Design review of the part built by this model. Coordinates are the model's own, in mm. Give positions to 0.01 mm unless a question says otherwise; leave off trailing zeros. Write each loop counter-clockwise with the first axis right and the second up, starting at its lowest first coordinate (ties: lowest second). Pieces come first, ordered by that corner, then holes. Notation, with made-up numbers: (40, 51) -> (61, 51) arc R15 cw to (61, 79) -> close; hole circle Ø6 at (59, 31.5). An arc over 180 degrees is marked (long way). Write each question's results on one line, items separated by ' | '. Start each with the question number.
(1) Take a section at C-C (z = -7). State the section outline as (x, y) points (3 decimals), plus the area to 3 significant figures.
(2) Take a section at A-A (z = 4.5). State the section outline as (x, y) points (3 decimals), plus the area to 3 significant figures.
(3) Clearance check with flat-ended pins moving along their axes: pin 1 (1.5 mm diameter, centred on y = 1.5, z = -0.5, fed in from -X) (3 decimals); pin 2 (1 mm diameter, centred on x = -78.5, y = 2.5, fed in from -Z). State where each tip first meets the part, or that it passes through.
(4) Take a section at D-D (x = 24). State the section outline as (y, z) points (3 decimals).
(5) To check wall thickness, follow probe 1 along X at (y, z) = (0.65, 0.5) (3 decimals); probe 2 along X at (y, z) = (2.45, -9); probe 3 along Z at (x, y) = (-58, 1.45). State the ranges of each line that lie inside material, in increasing order.
(6) Take a section at B-B (y = 1.6). State the section outline as (x, z) points (3 decimals), plus the area to 3 significant figures.
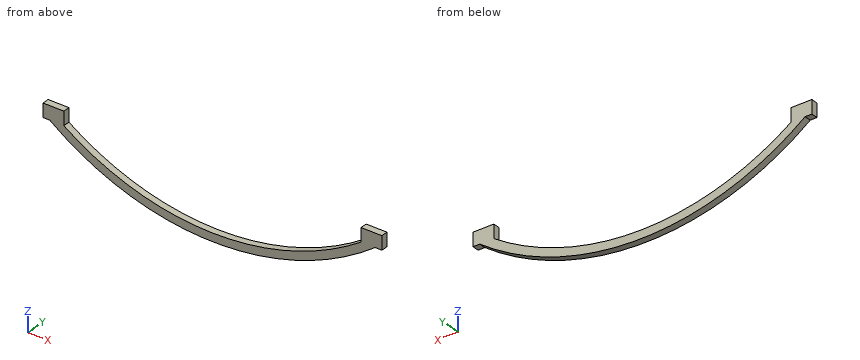
from build123d import *

# Parameters (mm, degrees)
BOSS_EXTRUDE2_DEPTH = 3.175
SKETCH2_W           = 9.745232509
SKETCH2_H           = 3.175
BOSS_EXTRUDE3_DEPTH = 6.35


with BuildPart() as part:
    # Sketch1 → Boss-Extrude2 (new body)
    with BuildSketch(Plane(origin=(0, 0, 0), x_dir=(1, 0, 0), z_dir=(0, 1, 0))):
        with BuildLine():
            Line((-76.2, 0), (-69.629767491, 0))
            ThreePointArc((-69.629767491, 0), (0, 21.43), (69.629767491, 0))
            Line((69.629767491, 0), (76.2, 0))
            ThreePointArc((76.2, 0), (0, 25.24), (-76.2, 0))
        make_face()
    extrude(amount=BOSS_EXTRUDE2_DEPTH)

    # Sketch2 → Boss-Extrude3 (add)
    with BuildSketch(Plane.XY):
        with Locations((-74.502383745, 1.5875)):
            Rectangle(SKETCH2_W, SKETCH2_H)
        with Locations((74.502383745, 1.5875)):
            Rectangle(SKETCH2_W, SKETCH2_H)
    extrude(amount=BOSS_EXTRUDE3_DEPTH)


solid = part.part
Report:
1) outline: (-65.755, 0) -> (-58.014, 0) -> (-58.014, 3.175) -> (-65.755, 3.175) -> close; (58.014, 0) -> (65.755, 0) -> (65.755, 3.175) -> (58.014, 3.175) -> close | area: 49.2 mm2
2) outline: (-79.375, 0) -> (-69.63, 0) -> (-69.63, 3.175) -> (-79.375, 3.175) -> close; (69.63, 0) -> (79.375, 0) -> (79.375, 3.175) -> (69.63, 3.175) -> close | area: 61.9 mm2
3) pin 1: x = -79.375 | pin 2: z = 0
4) outline: (0, -22.963) -> (3.175, -22.963) -> (3.175, -19.082) -> (0, -19.082) -> close
5) probe 1: -79.375 to -69.63, 69.63 to 79.375 | probe 2: -62.31 to -54.07, 54.07 to 62.31 | probe 3: -11.3 to -7.01
6) outline: (-79.375, 0) -> (-76.2, 0) arc R127.645 ccw to (76.2, 0) -> (79.375, 0) -> (79.375, 6.35) -> (69.63, 6.35) -> (69.63, 0) arc R123.835 cw to (-69.63, 0) -> (-69.63, 6.35) -> (-79.375, 6.35) -> close | area: 717 mm2
